Source: three-view drawing plus pictorial views. Frame: mm from the lowest corner of the part. A direction names the side the tool comes from. Coordinates: 2 decimals unless noted, no trailing zeros. Write each loop counter-clockwise with the first axis right and the second up, starting at its lowest first coordinate (ties: lowest second). Pieces come first, ordered by that corner, then holes. Notation, with made-up numbers: (63.25, 67.5) -> (75.25, 67.5) arc R31 cw to (75.25, 96.5) -> close; hole circle Ø5 at (10, -8.5). An arc over 180 degrees is marked (long way). Write item = value, one per line.
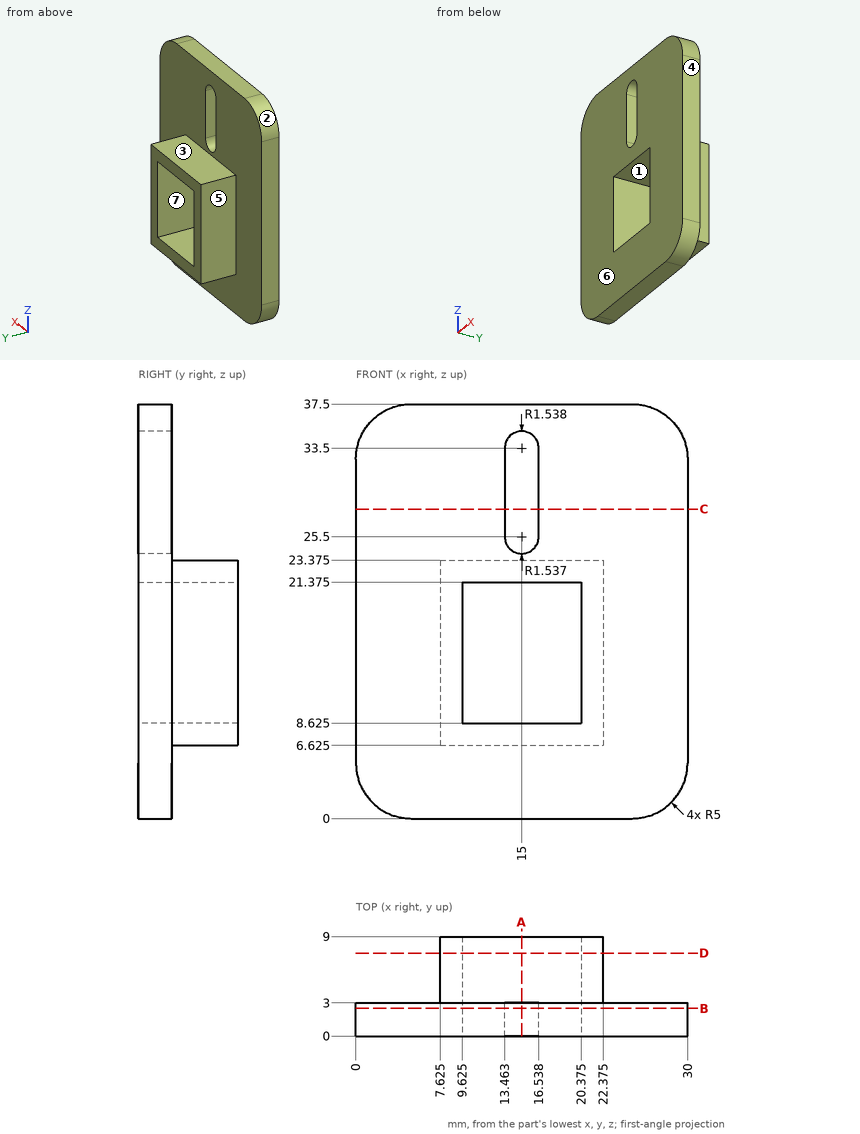
1) Reachability of the marked faces 5, 6 and 7 from +Z, -Z, +X, -X, +Y, -Y: full face, straight path, thin tool, end or side. Return the list, or none.
Answer block:
face_5 = +Z, -Z, -X, +Y
face_6 = +Z, -Z, +X, -X, -Y
face_7 = +Y, -Y
2) Cut plane C-C, the plane z = 28. Output: boundary loops of the cut face in (x, y).
Answer block:
outline = (0, 0) -> (13.46, 0) -> (13.46, 3) -> (0, 3) -> close; (16.54, 0) -> (30, 0) -> (30, 3) -> (16.54, 3) -> close
3) Material intervals for probe 1 along X at (y, z) = (8, 9) (1 decimal); probe 2 along Z at (x, y) = (18.75, 2.5) (1 decimal); probe 3 along Z at (x, y) = (17.25, 4.75) (1 decimal), sorted ascending. Write a range as [from, to].
Answer block:
probe_1 = [7.6, 9.6], [20.4, 22.4]
probe_2 = [0, 8.6], [21.4, 37.5]
probe_3 = [6.6, 8.6], [21.4, 23.4]
4) Pull-direction query (X, two-part tool) for the marked faces 1, 2, 3 and 4; classes: +X half, -X half, draft (parallel to the pull), parting line (faces both ways), or undercut.
Answer block:
face_1 = undercut
face_2 = -X half
face_3 = draft
face_4 = +X half
5) Cut plane A-A, the plane x = 15. Output: boundary loops of the cut face in (y, z) (1 decimal).
Answer block:
outline = (0, 0) -> (3, 0) -> (3, 6.6) -> (9, 6.6) -> (9, 8.6) -> (0, 8.6) -> close; (0, 21.4) -> (9, 21.4) -> (9, 23.4) -> (3, 23.4) -> (3, 24) -> (0, 24) -> close; (0, 35) -> (3, 35) -> (3, 37.5) -> (0, 37.5) -> close
6) Cut plane B-B, the plane y = 2.5. Output: boundary loops of the cut face in (x, z) (1 decimal).
Answer block:
outline = (0, 5) arc R5 ccw to (5, 0) -> (25, 0) arc R5 ccw to (30, 5) -> (30, 32.5) arc R5 ccw to (25, 37.5) -> (5, 37.5) arc R5 ccw to (0, 32.5) -> close; hole (9.6, 8.6) -> (20.4, 8.6) -> (20.4, 21.4) -> (9.6, 21.4) -> close; hole (13.5, 25.5) arc R1.5 ccw to (16.5, 25.5) -> (16.5, 33.5) arc R1.5 ccw to (13.5, 33.5) -> close
7) First-contact query: pin 1 Ø4 at (x, y) = (18.5, 6) entering from +Z (1 decimal); pin 2 Ø1 at (y, z) = (4.5, 24) entering from +X; pin 3 Ø1.8 at (y, z) = (6.5, 16) entering from -X (1 decimal); pin 4 Ø3 at (x, y) = (16, 7) entering from -Z (1 decimal). Flat tips, straight axial feed; report the tip coordinate or a pass-through.
Answer block:
pin_1 = 23.4
pin_2 = through
pin_3 = 7.6
pin_4 = 6.6
8) Cut plane D-D, the plane y = 7.5. Output: boundary loops of the cut face in (x, z) (1 decimal), and give its area (3 significant figures).
Answer block:
outline = (7.6, 6.6) -> (22.4, 6.6) -> (22.4, 23.4) -> (7.6, 23.4) -> close; hole (9.6, 8.6) -> (20.4, 8.6) -> (20.4, 21.4) -> (9.6, 21.4) -> close
area = 110 mm2
